Design review of the part built by this model. Coordinates are the model's own, in mm. Face numbers are marked on the shaded views. A direction names the side the tool comes from. Give positions to 0.01 mm unless a question says otherwise; leave off trailing zeros. Loops run counter-clockwise (first coordinate to the right, second up) from the corner with the lowest first, then second, coordinate; pieces in that order, holes last.
from build123d import *

# Parameters (mm, degrees)
SKETCH1_W           = 100
SKETCH1_H           = 54
BOSS_EXTRUDE1_DEPTH = 3
SKETCH2_W           = 76
SKETCH2_H           = 3
BOSS_EXTRUDE2_DEPTH = 10
CHAMFER1_SIZE       = 10
SKETCH3_W           = 10
SKETCH3_H           = 10
CUT_EXTRUDE1_DEPTH  = 10
SKETCH4_R           = 1.55
CUT_EXTRUDE2_DEPTH  = 3


with BuildPart() as part:
    # Sketch1 → Boss-Extrude1 (new body)
    with BuildSketch(Plane(origin=(0, 0, 0), x_dir=(1, 0, 0), z_dir=(0, 1, 0))):
        Rectangle(SKETCH1_W, SKETCH1_H)
    extrude(amount=BOSS_EXTRUDE1_DEPTH)

    # Sketch2 → Boss-Extrude2 (add)
    with BuildSketch(Plane.XZ):
        with Locations((0, 22.4)):
            Rectangle(SKETCH2_W, SKETCH2_H)
        with Locations((0, -22.4)):
            Rectangle(SKETCH2_W, SKETCH2_H)
    extrude(amount=BOSS_EXTRUDE2_DEPTH)

    # Chamfer1
    chamfer1_edges = [part.edges().sort_by_distance(p)[0] for p in [
        (0, 0, -20.9),
        (0, 0, 20.9),
    ]]
    chamfer(chamfer1_edges, length=CHAMFER1_SIZE - 0.0001)  # a hair under: the kernel refuses the full size

    # Sketch3 → Cut-Extrude1 (cut)
    with BuildSketch(Plane.XZ.offset(10)):
        with Locations((-20, 15.9)):
            Rectangle(SKETCH3_W, SKETCH3_H)
        with Locations((20, 15.9)):
            Rectangle(SKETCH3_W, SKETCH3_H)
    extrude(amount=-CUT_EXTRUDE1_DEPTH, mode=Mode.SUBTRACT)

    # Sketch4 → Cut-Extrude2 (cut)
    with BuildSketch(Plane.XY.offset(23.9)):
        with Locations((-20, -5)):
            Circle(SKETCH4_R)
        with Locations((20, -5)):
            Circle(SKETCH4_R)
    extrude(amount=-CUT_EXTRUDE2_DEPTH, mode=Mode.SUBTRACT)


solid = part.part
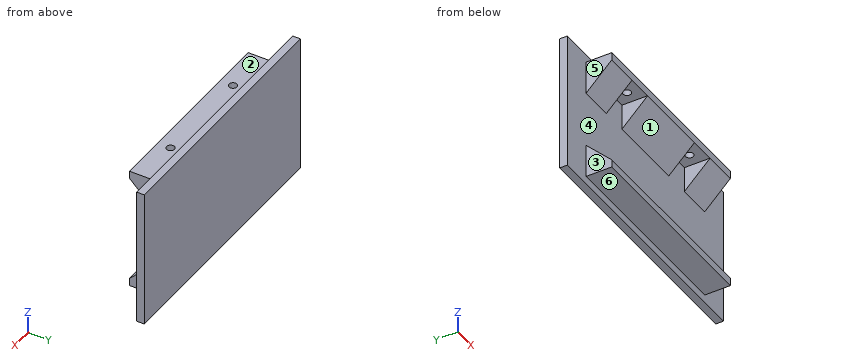
Q1. Take a section at C-C (z = -18). Give the boundary of the cut face in (x, y).
Results:
outline: (-50, 0) - (-38, 0) - (-38, -7.1) - (38, -7.1) - (38, 0) - (50, 0) - (50, 3) - (-50, 3) - close
Q2. Insertion check: pin 1 (1.5 mm diameter, centred on x = -21, z = -16, fed in from -Y); pin 2 (3 mm diameter, centred on x = 24.5, y = -3.5, fed in from -Z); pin 3 (3 mm diameter, centred on y = -4.5, z = 17.5, fed in from -X). Each pin has a flat end and moves straight along its axis. Give the tip position at first contact, or say it passes through.
Results:
pin 1: stops at y = -5.85
pin 2: stops at z = -23.9
pin 3: stops at x = -38
Q3. Tool access review of the marked faces 1, 2 and 3: name each direction out of +Z, -Z, +X, -X, +Y, -Y from which nothing blocks a thin tool from reaching the whole face with its end or side.
Results:
face 1: +X, -X, -Y
face 2: +Z, +X, -X, -Y
face 3: +Z, -Z, -X, -Y
Q4. Draft analysis for pull direction Z (two halves, no side actions). For the marked faces 4, 5 and 6, state which applies: pulls with the +Z half, pulls with the -Z half, needs draft (parallel to the pull), parting line crosses it, or undercut.
Results:
face 4: undercut
face 5: needs draft
face 6: pulls with the -Z half
Q5. Take a section at D-D (z = 2). Give the boundary of the cut face in (x, y).
Results:
outline: (-50, 0) - (50, 0) - (50, 3) - (-50, 3) - close
Q6. Take a section at B-B (y = -5). Give the boundary of the cut face in (x, z), plus the area to 3 significant figures.
Results:
outline: (-38, -23.9) - (38, -23.9) - (38, -15.9) - (-38, -15.9) - close; (-38, 15.9) - (-25, 15.9) - (-25, 20.9) - (-21.55, 20.9) - (-21.55, 23.9) - (-38, 23.9) - close; (-18.45, 20.9) - (-15, 20.9) - (-15, 15.9) - (15, 15.9) - (15, 20.9) - (18.45, 20.9) - (18.45, 23.9) - (-18.45, 23.9) - close; (21.55, 20.9) - (25, 20.9) - (25, 15.9) - (38, 15.9) - (38, 23.9) - (21.55, 23.9) - close
area: 1,100 mm2
Q7. Wall thickness on line 1 (X direction, y = -3.25, z = 18); line 2 (Y direction, x = 20, z = 21.6); line 3 (X direction, y = -3.75, z = 22): over which ranges is each line inside the solid? List them lowest first.
Results:
line 1: x = -38 to -25, -15 to 15, 25 to 38
line 2: y = -10 to -6.55, -3.45 to 3
line 3: x = -38 to -20.92, -19.08 to 19.08, 20.92 to 38
